Part model, mm, in its own coordinate system. A direction names the side the tool comes from. Round coordinates to 2 decimals unless told otherwise and drop trailing zeros. Loops run counter-clockwise (first coordinate to the right, second up) from the corner with the lowest first, then second, coordinate; pieces in that order, holes last.
1) Probe line 1 (Z direction, x = 2.5, y = 2.5); line 2 (X direction, y = 2.5, z = 22); line 3 (X direction, y = -2.25, z = 17). List the from-to ranges inside material, lowest first.
2) Mould opens along Z. For faces 1 (the cylindrical face through (0, -2, 2)), 2 (the cylindrical face through (-0.54, -2.44, 11.92)), 3 (the flat face through (2, -2, 4)) say: +Z half, -Z half, draft (parallel to the pull), parting line (faces both ways), or undercut.
3) Band-saw the part on B-B, the plane z = 3.5. Write the cut outline in (x, y).
4) Band-saw the part on A-A, the plane z = 11. Write the cut outline in (x, y), then the cut area to 3 significant figures.
5) Drop flat-ended pins along their axis: P1, Ø2, axis at x = 0.5, z = 0, coming from the +Y side; P2, Ø3, axis at x = -2, y = 1, coming from the -Z side; P3, Ø1, axis at y = 4, z = 18, coming from the +X side; P4, Ø3, axis at x = 1.5, y = -4, coming from the +Z side. Give the stop position or say it passes through.
6) 3-axis set-ups, long thin cutter, end or side, ignore diameter. For faces 4 (the cylindrical face through (0, -2, -3)), 5 (the cylindrical face through (-1.19, -5.37, 18.74)), 6 (the flat face through (0, 3, 6)): which of +Z, -Z, +X, -X, +Y, -Y reach the whole face in a straight line?
from build123d import *

# Parameters (mm, degrees)
SKETCH1_R           = 2
BOSS_EXTRUDE1_DEPTH = 4
SKETCH2_R           = 3.75
BOSS_EXTRUDE2_DEPTH = 2
SKETCH3_R           = 2.5
BOSS_EXTRUDE3_DEPTH = 12
SKETCH4_R           = 5.5
BOSS_EXTRUDE4_DEPTH = 6.5
FILLET1_R           = 5
SKETCH5_R           = 1.6
BOSS_EXTRUDE5_DEPTH = 1
SKETCH6_R           = 2
BOSS_EXTRUDE6_DEPTH = 5
FILLET2_R           = 0.3


with BuildPart() as part:
    # Sketch1 → Boss-Extrude1 (new body)
    with BuildSketch(Plane.XY):
        Circle(SKETCH1_R)
    extrude(amount=BOSS_EXTRUDE1_DEPTH)

    # Sketch2 → Boss-Extrude2 (add)
    with BuildSketch(Plane.XY.offset(4)):
        Circle(SKETCH2_R)
    extrude(amount=BOSS_EXTRUDE2_DEPTH)

    # Sketch3 → Boss-Extrude3 (add)
    with BuildSketch(Plane.XY.offset(6)):
        Circle(SKETCH3_R)
    extrude(amount=BOSS_EXTRUDE3_DEPTH)

    # Sketch4 → Boss-Extrude4 (add)
    with BuildSketch(Plane.XY.offset(18)):
        Circle(SKETCH4_R)
    extrude(amount=BOSS_EXTRUDE4_DEPTH)

    # Fillet1
    fillet1_edges = [part.edges().sort_by_distance(p)[0] for p in [
        (-5.5, 0, 24.5),
    ]]
    fillet(fillet1_edges, radius=FILLET1_R)

    # Sketch5 → Boss-Extrude5 (add)
    with BuildSketch(Plane(origin=(0, 0, 0), x_dir=(-1, 0, 0), z_dir=(0, 0, -1))):
        Circle(SKETCH5_R)
    extrude(amount=BOSS_EXTRUDE5_DEPTH)

    # Sketch6 → Boss-Extrude6 (add)
    with BuildSketch(Plane(origin=(0, 0, -1), x_dir=(-1, 0, 0), z_dir=(0, 0, -1))):
        Circle(SKETCH6_R)
    extrude(amount=BOSS_EXTRUDE6_DEPTH)

    # Fillet2
    fillet2_edges = [part.edges().sort_by_distance(p)[0] for p in [
        (1.6, 0, 0),
        (1.6, 0, -1),
    ]]
    fillet(fillet2_edges, radius=FILLET2_R)


solid = part.part
Reported:
1. line 1: z = 4 to 6, 18 to 23.47
1. line 2: x = -4.13 to 4.13
1. line 3: x = -1.09 to 1.09
2. face 1: draft
2. face 2: undercut
2. face 3: -Z half
3. outline: circle Ø4 at (0, 0)
4. outline: circle Ø5 at (0, 0)
4. area: 19.6 mm2
5. P1: stops at y = 2
5. P2: stops at z = -6
5. P3: stops at x = 4.24
5. P4: stops at z = 23.95
6. face 4: -Z
6. face 5: +Z, -Z
6. face 6: none
